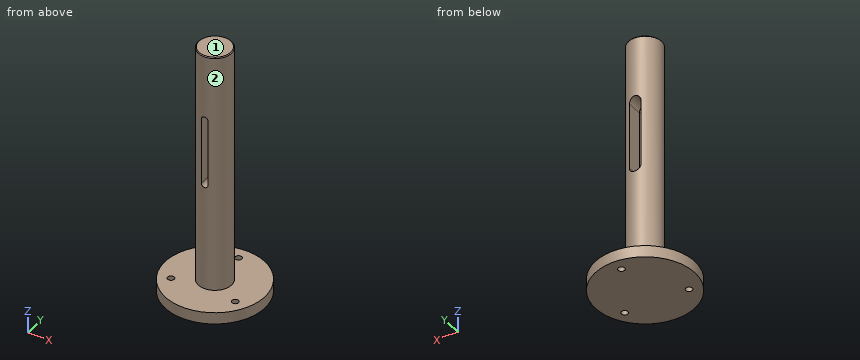
```python
from build123d import *

# Parameters (mm, degrees)
SKETCH1_R               = 30
SKETCH1_R_2             = 2
BOSS_EXTRUDE1_DEPTH     = 7
SKETCH2_R               = 10
BOSS_EXTRUDE2_DEPTH     = 145
CUT_EXTRUDE1_DEPTH      = 25
CUT_EXTRUDE1_DEPTH_BACK = 1.5
CHAMFER2_SIZE           = 1.5
CUT_EXTRUDE2_DEPTH      = 25
CHAMFER1_SIZE           = 0.5


with BuildPart() as part:
    # Sketch1 → Boss-Extrude1 (new body)
    with BuildSketch(Plane.XY):
        Circle(SKETCH1_R)
        with Locations((0, 22.5)):
            Circle(SKETCH1_R_2, mode=Mode.SUBTRACT)
        with Locations((19.485571585, -11.25)):
            Circle(SKETCH1_R_2, mode=Mode.SUBTRACT)
        with Locations((-19.485571585, -11.25)):
            Circle(SKETCH1_R_2, mode=Mode.SUBTRACT)
    extrude(amount=BOSS_EXTRUDE1_DEPTH)

    # Sketch2 → Boss-Extrude2 (add)
    with BuildSketch(Plane.XY.offset(7)):
        Circle(SKETCH2_R)
    extrude(amount=BOSS_EXTRUDE2_DEPTH)

    # Sketch3 → Cut-Extrude1 (cut, two sides)
    with BuildSketch(Plane(origin=(0, 0, 0), x_dir=(1, 0, 0), z_dir=(0, 1, 0))) as cut_extrude1_sk:
        with BuildLine():
            Line((3.5, -72), (3.5, -112))
            ThreePointArc((3.5, -112), (0, -115.5), (-3.5, -112))
            Line((-3.5, -112), (-3.5, -72))
            ThreePointArc((-3.5, -72), (0, -68.5), (3.5, -72))
        make_face()
    extrude(amount=CUT_EXTRUDE1_DEPTH, mode=Mode.SUBTRACT)
    extrude(cut_extrude1_sk.sketch, amount=-CUT_EXTRUDE1_DEPTH_BACK, mode=Mode.SUBTRACT)

    # Chamfer2
    chamfer2_edges = [part.edges().sort_by_distance(p)[0] for p in [
        (0, -1.5, 68.5),
        (3.5, -1.5, 92),
        (0, -1.5, 115.5),
        (-3.5, -1.5, 92),
    ]]
    chamfer(chamfer2_edges, length=CHAMFER2_SIZE)

    # Sketch4 → Cut-Extrude2 (cut)
    with BuildSketch(Plane(origin=(0, 0, 0), x_dir=(1, 0, 0), z_dir=(0, 1, 0))):
        with BuildLine():
            Line((2, -72), (2, -112))
            ThreePointArc((2, -112), (0, -114), (-2, -112))
            Line((-2, -112), (-2, -72))
            ThreePointArc((-2, -72), (0, -70), (2, -72))
        make_face()
    extrude(amount=-CUT_EXTRUDE2_DEPTH, mode=Mode.SUBTRACT)

    # Chamfer1
    chamfer1_edges = [part.edges().sort_by_distance(p)[0] for p in [
        (-10, 0, 152),
    ]]
    chamfer(chamfer1_edges, length=CHAMFER1_SIZE)


solid = part.part
```
CAD build for the part. Positions are in the model's coordinates, mm. Face numbers are marked on the shaded views. A direction names the side the tool comes from. Coordinates: 2 decimals unless noted, no trailing zeros. Loops run counter-clockwise (first coordinate to the right, second up) from the corner with the lowest first, then second, coordinate; pieces in that order, holes last. Notation, with made-up numbers: (-18, 56) - (-3, 56) arc R25 ccw to (-3, 84) - close; hole circle Ø7 at (-26, 81.5). An arc over 180 degrees is marked (long way). Return JSON: item names as keys, results as strings.
1. Probe L1, parallel to Y at x = 0, z = 5.75; L2, parallel to Z at x = -7.5, y = -23.5; L3, parallel to X at y = -8, z = 81. List the from-to ranges inside material, lowest first. Write a range as from..to.
Result:
{"L1": "y = -30..20.5, 24.5..30", "L2": "z = 0..7", "L3": "x = -6..-2, 2..6"}
2. Band-saw the part on D-D (z = 134). Give the cut face in (x, y), and give its area (3 significant figures).
Result:
{"outline": "circle Ø20 at (0, 0)", "area": "314 mm2"}
3. Band-saw the part on B-B (x = 0). Give the cut face in (y, z), and give its area (3 significant figures).
Result:
{"outline": "(-30, 0) - (20.5, 0) - (20.5, 7) - (10, 7) - (10, 68.5) - (0, 68.5) - (-1.5, 70) - (-10, 70) - (-10, 7) - (-30, 7) - close; (-10, 114) - (-1.5, 114) - (0, 115.5) - (10, 115.5) - (10, 151.5) - (9.5, 152) - (-9.5, 152) - (-10, 151.5) - close; (24.5, 0) - (30, 0) - (30, 7) - (24.5, 7) - close", "area": "2,380 mm2"}
4. Band-saw the part on A-A (z = 104.5). Give the cut face in (x, y), and give its area (3 significant figures).
Result:
{"outline": "(-3.5, 0) - (-3.5, 9.37) arc R10 ccw to (-2, -9.8) - (-2, -1.5) - close; (2, -9.8) arc R10 ccw to (3.5, 9.37) - (3.5, 0) - (2, -1.5) - close", "area": "204 mm2"}
5. Band-saw the part on C-C (y = 22.5). Give the cut face in (x, z), and give its area (3 significant figures).
Result:
{"outline": "(-19.84, 0) - (-2, 0) - (-2, 7) - (-19.84, 7) - close; (2, 0) - (19.84, 0) - (19.84, 7) - (2, 7) - close", "area": "250 mm2"}
6. 3-axis set-ups, long thin cutter, end or side, ignore diameter. For the marked faces 1 and 2: which of +Z, -Z, +X, -X, +Y, -Y reach the whole face in a straight line?
Result:
{"face 1": "+Z, +X, -X, +Y, -Y", "face 2": "+Z"}
7. Drop flat-ended pins along their axis: pin 1 (3 mm diameter, centred on x = -1.5, z = 77.5, fed in from -Y); pin 2 (9 mm diameter, centred on y = -4, z = 98, fed in from -X); pin 3 (3 mm diameter, centred on y = -6, z = 46.5, fed in from +X); pin 4 (4 mm diameter, centred on x = 23.5, y = 1.5, fed in from -Z). Give the stop position or say it passes through.
Result:
{"pin 1": "stops at y = -9.8", "pin 2": "stops at x = -10", "pin 3": "stops at x = 8.93", "pin 4": "stops at z = 0"}
